Input: dimensioned drawing with shaded views. Units: mm. Origin: part minimum x, y, z. A direction names the side the tool comes from. Round coordinates to 2 decimals unless told otherwise and drop trailing zeros. Loops run counter-clockwise (first coordinate to the right, second up) from the corner with the lowest first, then second, coordinate; pieces in that order, holes last. Notation, with made-up numbers: (-27.5, 75.25) - (-14.5, 75.25) arc R21 ccw to (-14.5, 88.25) - close; hole circle Ø7 at (78.25, 66.5). An arc over 180 degrees is marked (long way). Use CSV: the item, a comma, the result in double quotes. Start each with the question number.
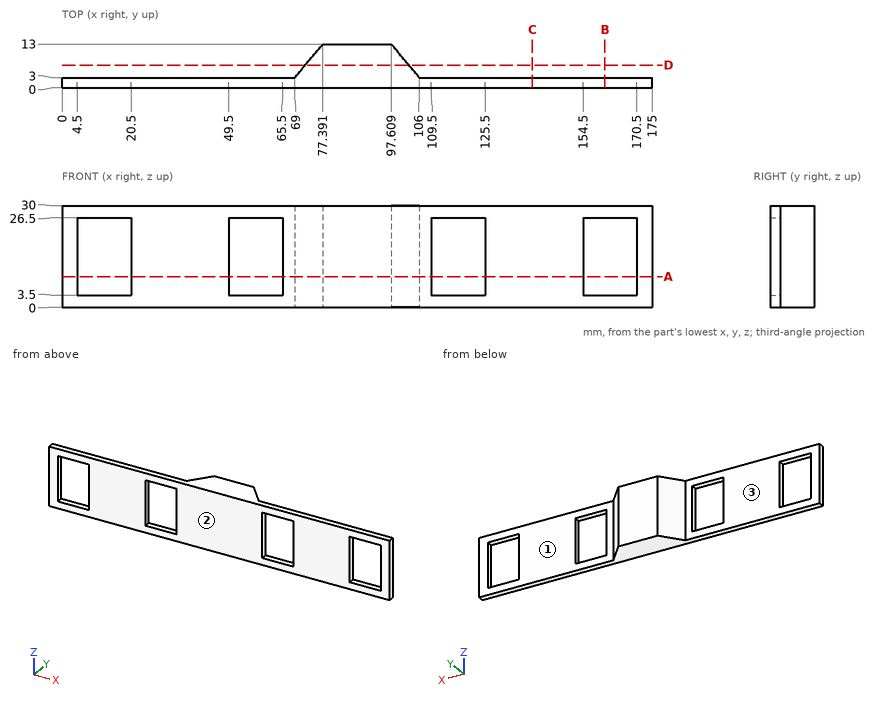
1. Section query C-C on x = 139.5. Return the cut outline in (y, z), and give its area (3 significant figures).
2. Reachability of the marked faces 1, 2 and 3 from +Z, -Z, +X, -X, +Y, -Y: full face, straight path, thin tool, end or side. Return the list, or none.
3. Section query A-A on z = 9. Give the number of separate pieces and of enclosed holes in the cut face, and give its area (3 significant figures).
4. Contact query for flat-ended pins moving along their axis: P1, Ø1.5, axis at y = 5, z = 15.5, coming from the +X side; P2, Ø3, axis at x = 35.5, z = 4, coming from the +Y side. Output: stop coordinate, or through.
5. Section query D-D on y = 6.75. Return the cut outline in (x, z).
6. Line query: line 1 along X through (y, z) = (2, 10.5); line 2 along Y through (x, z) = (21.5, 1.5); line 3 along X through (y, z) = (5.5, 2.5). Output: solid intervals per line, ascending.
7. Section query B-B on x = 161. Return the cut outline in (y, z), and give its area (3 significant figures).
Values:
1,outline,"(0, 0) - (3, 0) - (3, 30) - (0, 30) - close"
1,area,"90.0 mm^2"
2,face 1,"+Z, -Z, +X, +Y"
2,face 2,"+Z, -Z, +X, -X, -Y"
2,face 3,"+Z, -Z, -X, +Y"
3,separate pieces,"5"
3,enclosed holes,"0"
3,area,"619 mm^2"
4,P1,"stops at x = 104.95"
4,P2,"stops at y = 3"
5,outline,"(72.15, 0) - (102.85, 0) - (102.85, 30) - (72.15, 30) - close"
6,line 1,"x = 0 to 4.5, 20.5 to 49.5, 65.5 to 109.5, 125.5 to 154.5, 170.5 to 175"
6,line 2,"y = 0 to 3"
6,line 3,"x = 71.1 to 103.9"
7,outline,"(0, 0) - (3, 0) - (3, 3.5) - (0, 3.5) - close; (0, 26.5) - (3, 26.5) - (3, 30) - (0, 30) - close"
7,area,"21.0 mm^2"
